Verification items for this drawing (mm, ordinates from the low corner). A direction names the side the tool comes from. Round coordinates to 2 decimals unless told otherwise and drop trailing zeros. Loops run counter-clockwise (first coordinate to the right, second up) from the corner with the lowest first, then second, coordinate; pieces in that order, holes last. Notation, with made-up numbers: (79, 53) - (132, 53) arc R20 cw to (132, 92) - close; hole circle Ø6 at (5.5, 66.5). An arc over 180 degrees is marked (long way). Put each result on its own line as item: value.
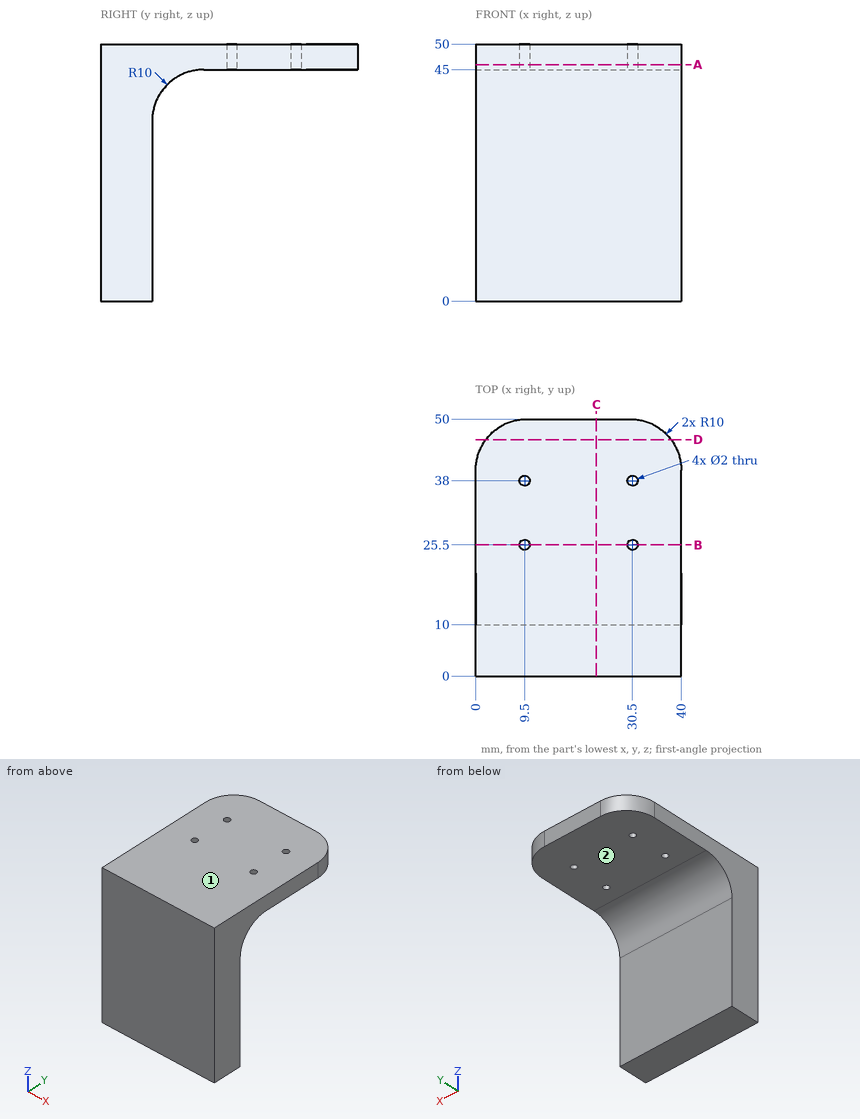
Item 1: Section check A-A on z = 46. Enter the section's corners in (x, y), then the cut area to 3 significant figures.
Filled sheet:
outline: (0, 0) - (40, 0) - (40, 40) arc R10 ccw to (30, 50) - (10, 50) arc R10 ccw to (0, 40) - close; hole circle Ø2 at (9.5, 25.5); hole circle Ø2 at (9.5, 38); hole circle Ø2 at (30.5, 25.5); hole circle Ø2 at (30.5, 38)
area: 1,940 mm²
Item 2: Section check B-B on y = 25.5. Enter the section's corners in (x, z).
Filled sheet:
outline: (0, 45) - (8.5, 45) - (8.5, 50) - (0, 50) - close; (10.5, 45) - (29.5, 45) - (29.5, 50) - (10.5, 50) - close; (31.5, 45) - (40, 45) - (40, 50) - (31.5, 50) - close
Item 3: Section check D-D on y = 46. Enter the section's corners in (x, z).
Filled sheet:
outline: (2, 45) - (38, 45) - (38, 50) - (2, 50) - close
Item 4: Tool access check on the marked faces 1 and 2. Record the directions out of +Z, -Z, +X, -X, +Y, -Y that give a thin tool (end or side, any length) a straight path to the whole face; none if there is none.
Filled sheet:
face 1: +Z, +X, -X, +Y, -Y
face 2: -Z, +X, -X, +Y
Item 5: Section check C-C on x = 23.5. Enter the section's corners in (y, z).
Filled sheet:
outline: (0, 0) - (10, 0) - (10, 35) arc R10 cw to (20, 45) - (50, 45) - (50, 50) - (0, 50) - close
Item 6: Go/stop test with flat-tipped pins: pin 1 (1.8 mm diameter, centred on x = 9.5, y = 38, fed in from -Z); pin 2 (1.5 mm diameter, centred on x = 35, z = 31.5, fed in from +Y); pin 3 (9 mm diameter, centred on x = 17.5, y = 27.5, fed in from -Z). Record where each tip stops, or that it passes through.
Filled sheet:
pin 1: through
pin 2: y = 10
pin 3: z = 45
Item 7: Thickness scan on line 1 (Y direction, x = 9.5, z = 47.25); line 2 (Y direction, x = 30, z = 46); line 3 (X direction, y = 25, z = 46). Record the ranges inside material, lowest first. Write a range as from..to.
Filled sheet:
line 1: 0..24.5, 26.5..37, 39..49.99
line 2: 0..24.63, 26.37..37.13, 38.87..50
line 3: 0..8.63, 10.37..29.63, 31.37..40
